Could you check a few things on this model? Use its own coordinates, in mm. Face numbers are marked on the shaded views. A direction names the side the tool comes from. Coordinates: 2 decimals unless noted, no trailing zeros. Order: outer loops, then holes, each group sorted by start corner. A loop starts at its lowest first (then second) coordinate and runs counter-clockwise, first axis right, second up. Notation, with made-up numbers: (19, 12.5) -> (72, 12.5) arc R38 ccw to (72, 50.5) -> close; hole circle Ø6 at (-16, 88.5). An arc over 180 degrees is marked (long way). Use a Markdown table: item, result. Add a question column.
1) If we section it at D-D (x = 51.5): Write out the boundary of the cut face in (y, z), plus the area to 3 significant figures.
2) If I drill on L1, parallel to X at y = -1, z = 4; L2, parallel to Y at x = -50, z = 4; L3, parallel to Z at x = -26, y = -22, over which ranges is the centre line in solid material (lowest first)? Write a range as [from, to].
3) If we section it at B-B (z = 7.5): Write out the boundary of the cut face in (x, y).
4) Thinking about a two-plate mould opening in Y: for the marked faces 1, 2 and 3, which applies, +Y half, -Y half, draft (parallel to the pull), parting line (faces both ways), or undercut?
5) Will these pins go through, and if not, where does the flat tip stop? pin 1 Ø7.5 at (x, z) = (-45, 5) entering from +Y; pin 2 Ø6 at (x, z) = (-15.5, 5) entering from -Y; pin 3 Ø10 at (y, z) = (17, -10) entering from -X.
6) If we section it at C-C (x = 0): Write out the boundary of the cut face in (y, z).
7) Which directions (+Z, -Z, +X, -X, +Y, -Y) give clear straight access to the entire face, cutting with the end or side of a thin tool? Please do the marked faces 4, 5, 6 and 7.
8) If we section it at A-A (y = 0): Give the number of separate pieces and of enclosed holes in the cut face, plus the area to 3 significant figures.
Autodesk Inventor part; units mm, degrees
ref_plane "YZ Plane" through (0, 0, 0) normal (1, 0, 0) x (0, 1, 0)
ref_plane "XZ Plane" through (0, 0, 0) normal (0, 1, 0) x (-1, 0, 0)
ref_plane "XY Plane" through (0, 0, 0) normal (0, 0, 1) x (1, 0, 0)
sketch "Sketch1" plane through (0, 0, 0) normal (0, 0, 1) x (1, 0, 0)
  arc A0 (50, -10) -> (50, 10) centre (50, 0) ccw
  arc A1 (-50, 10) -> (-50, -10) centre (-50, 0) ccw
  arc A2 (-43.3618, -10) -> (43.3618, -10) centre (0, 0) ccw
  arc A3 (43.3618, 10) -> (-43.3618, 10) centre (0, 0) ccw
  circle A4 centre (-50, 0) radius 3.5
  circle A5 centre (50, 0) radius 3.5
  line L0 (50, -10) -> (43.3618, -10)
  line L1 (-43.3618, -10) -> (-50, -10)
  line L2 (-50, 10) -> (-43.3618, 10)
  line L3 (43.3618, 10) -> (50, 10)
  dimension "d1" = 20
  dimension "d2" = 20
  dimension "d4" = 50
  dimension "d5" = 50
  dimension "d6" = 7
  dimension "d7" = 7
extrude "Extrusion1" add sketch "Sketch1" along normal blind 10
sketch "Sketch2" plane through (0, 0, 10) normal (0, 0, 1) x (1, 0, 0)
  circle A0 centre (0, 0) radius 36
  dimension "d10" = 72
extrude "Extrusion2" cut sketch "Sketch2" against normal blind 8
sketch "Sketch3" plane through (0, 0, 0) normal (0, 0, -1) x (-1, 0, 0)
  circle A0 centre (0, 0) radius 34.5
  dimension "d13" = 69
extrude "Extrusion3" add sketch "Sketch3" along normal blind 10
sketch "Sketch4" plane through (0, 0, -10) normal (0, 0, -1) x (-1, 0, 0)
  circle A0 centre (0, 0) radius 20
  dimension "d16" = 40
extrude "Extrusion4" add sketch "Sketch4" along normal blind 15
sketch "Sketch6" plane through (0, 0, 0) normal (0, 1, 0) x (-1, 0, 0)
  line L0 (-34.5, 0) -> (-34.5, -10)
  line L1 (-34.5, 0) -> (-34, 0)
  line L2 (-34, 0) -> (-34, -3)
  line L3 (-34, -3) -> (-34.5, -3)
  line L4 (-34.5, -3) -> (-34.5, 0)
  line L5 (-34.5, -10) -> (34.5, -10)
  line L6 (-20, -10) -> (-20, -25)
  line L7 (-20, -10) -> (-19.5, -10)
  line L8 (-19.5, -10) -> (-19.5, -15)
  line L9 (-19.5, -15) -> (-20, -15)
  line L10 (-20, -15) -> (-20, -10)
  line L11 (0, 12.5498) -> (0, -27.5159) construction
  point P0 (0, 0)
  dimension "d19" = 0.5
  dimension "d20" = 3
  dimension "d21" = 7
  dimension "d22" = 0.5
  dimension "d23" = 5
revolve "Revolution1" cut sketch "Sketch6" angle 360 about axis through (0, 0, 12.5498) along (0, 0, -1)
properties part number "Prato do Amassador"
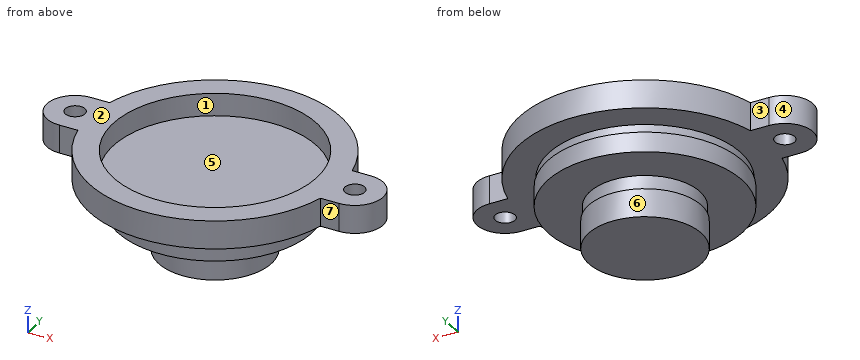
Answer sheet:
| question | item | result |
|---|---|---|
| 1 | outline | (-9.89, 0) -> (-3.16, 0) -> (-3.16, 10) -> (-9.89, 10) -> close; (3.16, 0) -> (9.89, 0) -> (9.89, 10) -> (3.16, 10) -> close |
| 1 | area | 134 mm2 |
| 2 | L1 | [-59.95, -53.35], [-46.65, -35.99], [35.99, 46.65], [53.35, 59.95] |
| 2 | L2 | [-10, -3.5], [3.5, 10] |
| 2 | L3 | [-10, -3], [0, 2] |
| 3 | outline | (-50, -10) -> (-43.36, -10) arc R44.5 ccw to (43.36, -10) -> (50, -10) arc R10 ccw to (50, 10) -> (43.36, 10) arc R44.5 ccw to (-43.36, 10) -> (-50, 10) arc R10 ccw to start; hole circle Ø7 at (-50, 0); hole circle Ø72 at (0, 0); hole circle Ø7 at (50, 0) |
| 4 | face 1 | undercut |
| 4 | face 2 | draft |
| 4 | face 3 | +Y half |
| 5 | pin 1 | y = 16.69 |
| 5 | pin 2 | y = -42.71 |
| 5 | pin 3 | x = -32.35 |
| 6 | outline | (-44.5, 0) -> (-34, 0) -> (-34, -3) -> (-34.5, -3) -> (-34.5, -10) -> (-19.5, -10) -> (-19.5, -15) -> (-20, -15) -> (-20, -25) -> (20, -25) -> (20, -15) -> (19.5, -15) -> (19.5, -10) -> (34.5, -10) -> (34.5, -3) -> (34, -3) -> (34, 0) -> (44.5, 0) -> (44.5, 10) -> (36, 10) -> (36, 2) -> (-36, 2) -> (-36, 10) -> (-44.5, 10) -> close |
| 7 | face 4 | +Z, -Z, -X |
| 7 | face 5 | +Z |
| 7 | face 6 | -Z |
| 7 | face 7 | +Z, -Z, +X, -Y |
| 8 | separate pieces | 3 |
| 8 | enclosed holes | 0 |
| 8 | area | 1,770 mm2 |
